from build123d import *

# Parameters (mm, degrees)
F0_R     = 1.15
F1_DEPTH = 3


with BuildPart() as f1:
    # F0 (on Right) → F1 (new body)
    with BuildSketch(Plane.YZ):
        with BuildLine():
            Line((-12, 0), (-12, 6))
            Line((-12, 6), (12, 6))
            Line((12, 6), (12, 0))
            Line((12, 0), (12, -6))
            Line((12, -6), (17, -6))
            Line((17, -6), (17, 8))
            ThreePointArc((17, 8), (16.12132, 10.12132), (14, 11))
            Line((14, 11), (0, 11))
            Line((0, 11), (-14, 11))
            ThreePointArc((-14, 11), (-16.12132, 10.12132), (-17, 8))
            Line((-17, 8), (-17, -6))
            Line((-17, -6), (-12, -6))
            Line((-12, -6), (-12, 0))
        make_face()
        with Locations((-13.8, 0)):
            Circle(F0_R, mode=Mode.SUBTRACT)
        with BuildLine():
            ThreePointArc((14.95, 0), (13.8, -1.15), (12.65, 0))
            ThreePointArc((12.65, 0), (13.8, 1.15), (14.95, 0))
        make_face(mode=Mode.SUBTRACT)
    extrude(amount=F1_DEPTH)


solid = f1.part
For this review, take the finished solid that the model builds, in its own axes (mm). A direction names the side the tool comes from. Round coordinates to 2 decimals unless told otherwise and drop trailing zeros. Order: outer loops, then holes, each group sorted by start corner. A loop starts at its lowest first (then second) coordinate and runs counter-clockwise, first axis right, second up. Notation, with made-up numbers: M 66.25,-14 L 75.25,-14 A21 cw 75.25,6 Z; hole C 32.5,-11.75 d1. An arc over 180 degrees is marked long. Use a Markdown table: item, result. Add a question column.
Item 1: Tool access review of faces 1 (the flat face through (1, -17, 1)), 2 (the flat face through (1, 0, 6)): name each direction out of +Z, -Z, +X, -X, +Y, -Y from which nothing blocks a thin tool from reaching the whole face with its end or side.
Item 2: Insertion check: pin 1 (1.5 mm diameter, centred on x = 2, y = -2.5, fed in from -Z); pin 2 (6 mm diameter, centred on y = -8, z = 1.5, fed in from +X). Each pin has a flat end and moves straight along its axis. Give the tip position at first contact, or say it passes through.
Item 3: To check wall thickness, follow line 1 along Z through (x, y) = (1.45, -13.8); line 2 along Y through (x, z) = (0.35, 3.75); line 3 along Z through (x, y) = (1.75, -4). State the ranges of each line that lie inside material, in increasing order.
Item 4: Add section A-A, the plane z = 4.5. Give the boundary of the cut face in (x, y), then the cut area to 3 significant figures.
Item 5: Add section B-B, the plane x = 2.1. Give the boundary of the cut face in (y, z).
Item 6: Add section D-D, the plane y = 9. Give the boundary of the cut face in (x, z), then the cut area to 3 significant figures.
Item 7: Add section C-C, the plane z = 0. Give the boundary of the cut face in (x, y).
Item 8: Mouldability with a two-part tool opening along Z and no side actions: class faces 3 (the cylindrical face through (1.479, -12.703, 0.345)), 4 (the cylindrical face through (1.479, 12.738, -0.44)), 5 (the flat face through (1, 0, 11)), 6 (the flat face through (1, -15, -6)) as released by +Z, released by -Z, zero draft, split by the parting line, or undercut.
Geometry results:
| question | item | result |
|---|---|---|
| 1 | face 1 | +Z, -Z, +X, -X, -Y |
| 1 | face 2 | -Z, +X, -X |
| 2 | pin 1 | stops at z = 6 |
| 2 | pin 2 | passes through |
| 3 | line 1 | z = -6 to -1.15, 1.15 to 11 |
| 3 | line 2 | y = -17 to -12, 12 to 17 |
| 3 | line 3 | z = 6 to 11 |
| 4 | outline | M 0,-17 L 3,-17 L 3,-12 L 0,-12 Z; M 0,12 L 3,12 L 3,17 L 0,17 Z |
| 4 | area | 30.0 mm² |
| 5 | outline | M -17,-6 L -12,-6 L -12,6 L 12,6 L 12,-6 L 17,-6 L 17,8 A3 ccw 14,11 L -14,11 A3 ccw -17,8 Z; hole C -13.8,0 d2.3; hole C 13.8,0 d2.3 |
| 6 | outline | M 0,6 L 3,6 L 3,11 L 0,11 Z |
| 6 | area | 15.0 mm² |
| 7 | outline | M 0,-17 L 3,-17 L 3,-14.95 L 0,-14.95 Z; M 0,-12.65 L 3,-12.65 L 3,-12 L 0,-12 Z; M 0,12 L 3,12 L 3,12.65 L 0,12.65 Z; M 0,14.95 L 3,14.95 L 3,17 L 0,17 Z |
| 8 | face 3 | undercut |
| 8 | face 4 | undercut |
| 8 | face 5 | released by +Z |
| 8 | face 6 | released by -Z |
